Autodesk Inventor part; units mm, degrees
ref_plane "YZ Plane" through (0, 0, 0) normal (1, 0, 0) x (0, 1, 0)
ref_plane "XZ Plane" through (0, 0, 0) normal (0, 1, 0) x (-1, 0, 0)
ref_plane "XY Plane" through (0, 0, 0) normal (0, 0, 1) x (1, 0, 0)
sketch "Szkic1" plane through (0, 0, 0) normal (0, 1, 0) x (-1, 0, 0)
  circle A0 centre (-0.3368, -8.6859) radius 3
  circle A1 centre (-0.3368, -1.6859) radius 3
  line L0 (3.6632, 2.3141) -> (-4.3368, 2.3141)
  line L1 (-4.3368, 2.3141) -> (-4.3368, -12.6859)
  line L2 (-4.3368, -12.6859) -> (3.6632, -12.6859)
  line L3 (3.6632, -12.6859) -> (3.6632, 2.3141)
  point P0 (0, 0)
  dimension "d0" = 6
  dimension "d1" = 6
  dimension "d2" = 7
  dimension "d3" = 8
  dimension "d4" = 15
  dimension "d5" = 4
  dimension "d6" = 4
extrude "Wyciągnięcie proste1" add sketch "Szkic1" along normal blind 10
fillet "Zaokrąglenie1" radius 2 4 edges at (4.3368, 5, 2.3141) (-3.6632, 5, 2.3141) (4.3368, 5, -12.6859) (-3.6632, 5, -12.6859)
properties part number "obudowa"
Design review of the part built by this model. Coordinates are the model's own, in mm. Coordinates: 2 decimals unless noted, no trailing zeros. Loops run counter-clockwise (first coordinate to the right, second up) from the corner with the lowest first, then second, coordinate; pieces in that order, holes last.
Q1. The part is to be moulded in two halves that separate along X. For faces 1 (the face through (3.77, 5.07, -12.08)), 2 (the face through (0, 0, -5)), 3 (the face through (-1, 5, 1)), say which applies: +X half, -X half, draft (parallel to the pull), parting line (faces both ways), or undercut.
Reported:
face 1: +X half
face 2: draft
face 3: undercut
Q2. To check wall thickness, follow line 1 (Z direction, x = 0.25, y = 5.5); line 2 (Z direction, x = -2, y = 5.25); line 3 (X direction, y = 7.25, z = -7.25). State the ranges of each line that lie inside material, in increasing order.
Reported:
line 1: z = -12.69 to -11.68, -5.69 to -4.68, 1.31 to 2.31
line 2: z = -12.66 to -10.57, -6.8 to -3.57, 0.2 to 2.29
line 3: x = -3.66 to -2.3, 2.97 to 4.34
Q3. We need section B-B on x = -2. State the section outline as (y, z) points.
Reported:
outline: (0, -12.66) - (10, -12.66) - (10, -10.57) - (0, -10.57) - close; (0, -6.8) - (10, -6.8) - (10, -3.57) - (0, -3.57) - close; (0, 0.2) - (10, 0.2) - (10, 2.29) - (0, 2.29) - close
Q4. We need section A-A on z = -11.5. State the section outline as (x, y) points.
Reported:
outline: (-3.49, 0) - (-0.7, 0) - (-0.7, 10) - (-3.49, 10) - close; (1.38, 0) - (4.16, 0) - (4.16, 10) - (1.38, 10) - close
Q5. We need section C-C on y = 4. State the section outline as (x, z) points, and give its area (3 significant figures).
Reported:
outline: (-3.66, -10.69) arc R2 ccw to (-1.66, -12.69) - (2.34, -12.69) arc R2 ccw to (4.34, -10.69) - (4.34, 0.31) arc R2 ccw to (2.34, 2.31) - (-1.66, 2.31) arc R2 ccw to (-3.66, 0.31) - close; hole circle Ø6 at (0.34, -8.69); hole circle Ø6 at (0.34, -1.69)
area: 60.0 mm2
Q6. We need section D-D on z = -4.5. State the section outline as (x, y) points, and give its area (3 significant figures).
Reported:
outline: (-3.66, 0) - (-0.7, 0) - (-0.7, 10) - (-3.66, 10) - close; (1.38, 0) - (4.34, 0) - (4.34, 10) - (1.38, 10) - close
area: 59.2 mm2
